The drawing under review shows one solid part. Ordinate dimensions are in mm from its lowest x, y, z. Give positions to 0.01 mm unless a question says otherwise; leave off trailing zeros. Loops run counter-clockwise (first coordinate to the right, second up) from the corner with the lowest first, then second, coordinate; pieces in that order, holes last. Notation, with made-up numbers: M -36,-37 L -14,-37 A22 cw -14,-28 Z; hole C 18,72.25 d3. An arc over 180 degrees is marked long. Put each result on its own line as item: value. Start each with the question number.
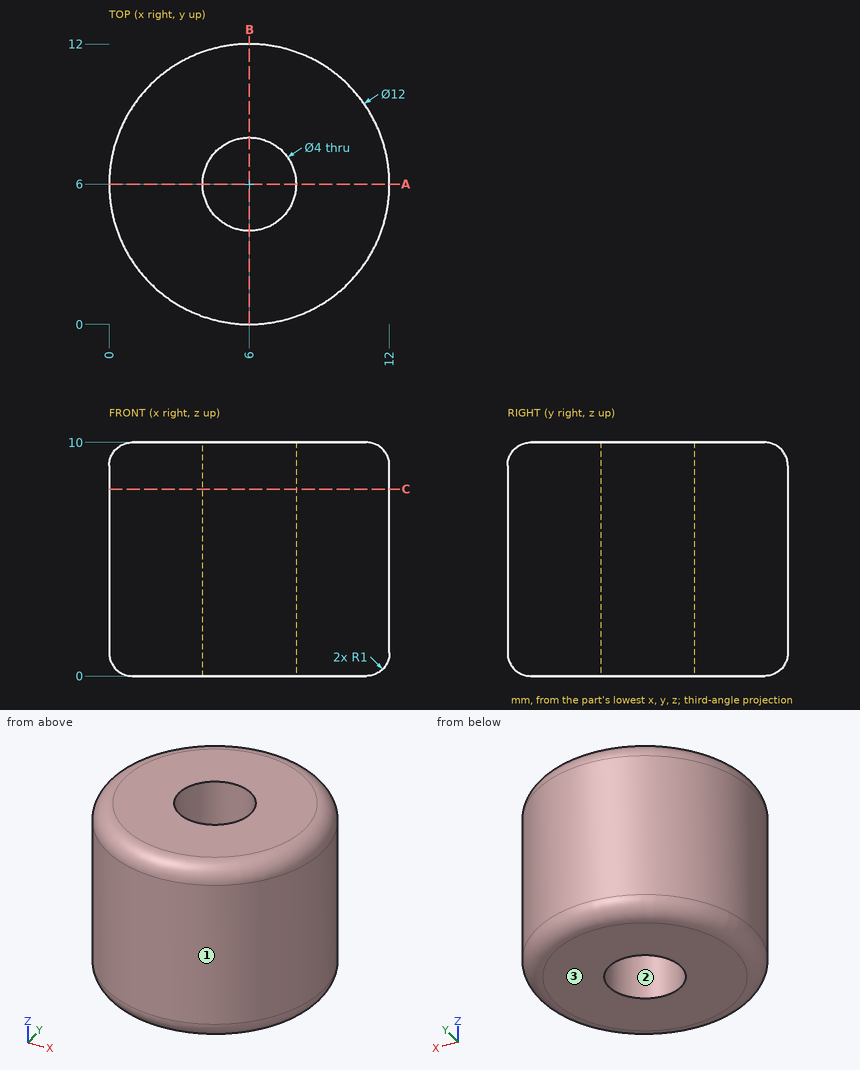
Item 1: Draft analysis for pull direction X (two halves, no side actions). For the marked faces 1, 2 and 3, state which applies: +X half, -X half, draft (parallel to the pull), parting line (faces both ways), or undercut.
Item 2: Clearance check with flat-ended pins moving along their axes: pin 1 Ø3 at (y, z) = (4, 8) entering from -X; pin 2 Ø4 at (x, z) = (3, 1.5) entering from +Y; pin 3 Ø3.5 at (x, y) = (6, 6) entering from +Z. State where each tip first meets the part, or that it passes through.
Item 3: Consider section A-A, the plane y = 6. Write out the cut boundary in (x, z).
Item 4: To check wall thickness, follow L1, parallel to Y at x = 6, z = 6.5; L2, parallel to X at y = 7.75, z = 8; L3, parallel to X at y = 5.75, z = 7.25. State the ranges of each line that lie inside material, in increasing order. Write a range as [from, to].
Item 5: Consider section C-C, the plane z = 8. Write out the cut boundary in (x, y), plus the area to 3 significant figures.
Report:
1. face 1: parting line
1. face 2: undercut
1. face 3: draft
2. pin 1: x = 0.02
2. pin 2: y = 11.92
2. pin 3: through
3. outline: M 0,1 A1 ccw 1,0 L 4,0 L 4,10 L 1,10 A1 ccw 0,9 Z; M 8,0 L 11,0 A1 ccw 12,1 L 12,9 A1 ccw 11,10 L 8,10 Z
4. L1: [0, 4], [8, 12]
4. L2: [0.26, 5.03], [6.97, 11.74]
4. L3: [0.01, 4.02], [7.98, 11.99]
5. outline: C 6,6 d12; hole C 6,6 d4
5. area: 101 mm²
